```python
from build123d import *

# Parameters (mm, degrees)
SKETCH1_R           = 9.525
BOSS_EXTRUDE1_DEPTH = 6.35
SKETCH2_R           = 2
CUT_EXTRUDE1_DEPTH  = 15.892070037
SKETCH5_R           = 14.2875
SKETCH5_R_2         = 2
BOSS_EXTRUDE3_DEPTH = 2.54
SKETCH6_R           = 14.2875
SKETCH6_R_2         = 2
BOSS_EXTRUDE4_DEPTH = 2.54
SKETCH7_R           = 0.79375
CUT_EXTRUDE2_DEPTH  = 24.214439741


with BuildPart() as part:
    # Sketch1 → Boss-Extrude1 (new body)
    with BuildSketch(Plane.XY):
        Circle(SKETCH1_R)
    extrude(amount=BOSS_EXTRUDE1_DEPTH)

    # Sketch2 → Cut-Extrude1 (cut, through all)
    with BuildSketch(Plane.XY.offset(6.35)):
        Circle(SKETCH2_R)
    extrude(amount=-CUT_EXTRUDE1_DEPTH, mode=Mode.SUBTRACT)

    # Sketch5 → Boss-Extrude3 (add)
    with BuildSketch(Plane.XY.offset(6.35)):
        Circle(SKETCH5_R)
        Circle(SKETCH5_R_2, mode=Mode.SUBTRACT)
    extrude(amount=BOSS_EXTRUDE3_DEPTH)

    # Sketch6 → Boss-Extrude4 (add)
    with BuildSketch(Plane(origin=(0, 0, 0), x_dir=(-1, 0, 0), z_dir=(0, 0, -1))):
        with Locations(Location((0, 0, 0), (0, 0, 180))):
            Circle(SKETCH6_R)
        with Locations(Location((0, 0, 0), (0, 0, 180))):
            Circle(SKETCH6_R_2, mode=Mode.SUBTRACT)
    extrude(amount=BOSS_EXTRUDE4_DEPTH)

    # Sketch7 → Cut-Extrude2 (cut, through all)
    with BuildSketch(Plane.XY.offset(8.89)):
        with Locations((0, 11.90625)):
            Circle(SKETCH7_R)
    extrude(amount=-CUT_EXTRUDE2_DEPTH, mode=Mode.SUBTRACT)


solid = part.part
```
The model under review builds one solid part; all positions refer to its coordinate system, in mm. A direction names the side the tool comes from. Give positions to 0.01 mm unless a question says otherwise; leave off trailing zeros. Write each loop counter-clockwise with the first axis right and the second up, starting at its lowest first coordinate (ties: lowest second). Pieces come first, ordered by that corner, then holes. Notation, with made-up numbers: (33.5, 47) - (52.5, 47) arc R20 cw to (52.5, 81) - close; hole circle Ø4 at (49.5, 48.5). An arc over 180 degrees is marked (long way). Answer in a Markdown table with one row per item. Add a question column.
1. Tool access review of faces 1 (the cylindrical face through (-14.274, 0.628, 7.602)), 2 (the cylindrical face through (-7.559, -5.796, 3.131)): name each direction out of +Z, -Z, +X, -X, +Y, -Y from which nothing blocks a thin tool from reaching the whole face with its end or side.
2. Wall thickness on line 1 along Y through (x, z) = (0, 7.95); line 2 along Z through (x, y) = (-8.5, -9); line 3 along Y through (x, z) = (1.5, -0.25): over which ranges is each line inside the solid? List them lowest first. Write a range as [from, to].
3. We need section C-C on z = 3. Write out the cut boundary in (x, y) (3 decimals), then the cut area to 3 significant figures.
4. We need section B-B on x = 0. State how many separate pieces and enclosed holes the cut face has, then the cut area to 3 significant figures.
5. We need section D-D on y = -12. Write out the cut boundary in (x, z), then the cut area to 3 significant figures.
6. Draft analysis for pull direction Z (two halves, no side actions). For faces 3 (the flat face through (9.3, 3, 0)), 4 (the flat face through (0, -3, 8.89)), 5 (the cylindrical face through (-14.274, -0.628, -1.252)), 6 (the flat face through (3, 0, -2.54)), state which applies: +Z half, -Z half, draft (parallel to the pull), parting line (faces both ways), or undercut.
7. Insertion check: P1, Ø3, axis at y = 7, z = 3, coming from the -X side; P2, Ø2, axis at y = 3.5, z = 3, coming from the -X side; P3, Ø1, axis at y = -5, z = 1.5, coming from the +X side (3 decimals). Each pin has a flat end and moves straight along its axis. Give the tip position at first contact, or say it passes through.
Ans:
| question | item | result |
|---|---|---|
| 1 | face 1 | +Z, -Z |
| 1 | face 2 | none |
| 2 | line 1 | y = [-14.29, -2], [2, 11.11], [12.7, 14.29] |
| 2 | line 2 | z = [-2.54, 0], [6.35, 8.89] |
| 2 | line 3 | y = [-14.21, -1.32], [1.32, 14.21] |
| 3 | outline | circle Ø19.05 at (0, 0); hole circle Ø4 at (0, 0) |
| 3 | area | 272 mm^2 |
| 4 | separate pieces | 4 |
| 4 | enclosed holes | 0 |
| 4 | area | 212 mm^2 |
| 5 | outline | (-7.75, -2.54) - (7.75, -2.54) - (7.75, 0) - (-7.75, 0) - close; (-7.75, 6.35) - (7.75, 6.35) - (7.75, 8.89) - (-7.75, 8.89) - close |
| 5 | area | 78.8 mm^2 |
| 6 | face 3 | undercut |
| 6 | face 4 | +Z half |
| 6 | face 5 | draft |
| 6 | face 6 | -Z half |
| 7 | P1 | stops at x = -7.78 |
| 7 | P2 | stops at x = -9.19 |
| 7 | P3 | stops at x = 8.395 |
